Part print with two shaded views. Sizes in mm from the minimum x, y, z corner. A direction names the side the tool comes from. Coordinates: 2 decimals unless noted, no trailing zeros. Loops run counter-clockwise (first coordinate to the right, second up) from the corner with the lowest first, then second, coordinate; pieces in that order, holes last. Notation, with made-up numbers: (50.25, -12.5) -> (105.25, -12.5) arc R19 cw to (105.25, 18.5) -> close; hole circle Ø9 at (26.5, -36.75). An arc over 180 degrees is marked (long way). Use one line per item in the form item = value.
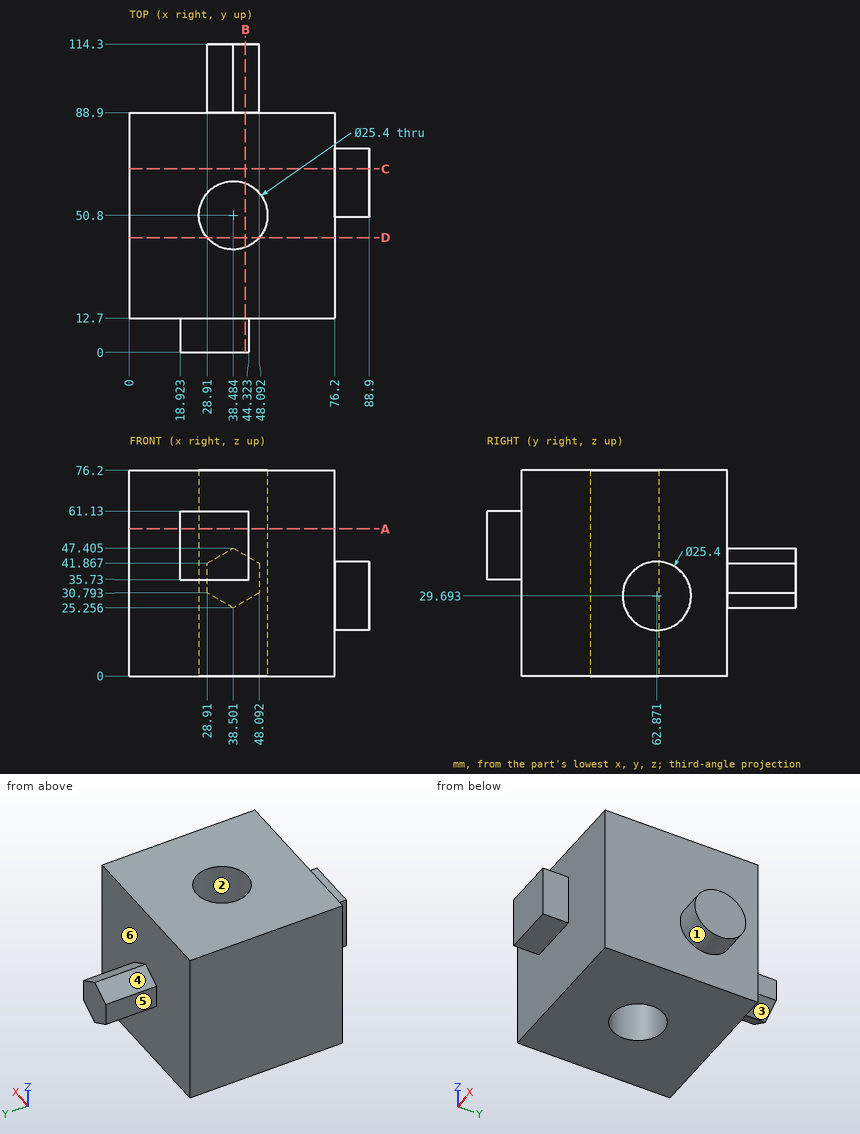
Q1. Mould opens along X. For the marked faces 1, 2 and 3 say: released by +X, released by -X, zero draft, split by the parting line, or undercut.
Result:
face_1 = zero draft
face_2 = undercut
face_3 = released by +X
Q2. Band-saw the part on B-B, the plane x = 43. Write the cut outline in (y, z).
Result:
outline = (0, 35.73) -> (12.7, 35.73) -> (12.7, 0) -> (38.93, 0) -> (38.93, 76.2) -> (12.7, 76.2) -> (12.7, 61.13) -> (0, 61.13) -> close; (62.67, 0) -> (88.9, 0) -> (88.9, 27.85) -> (114.3, 27.85) -> (114.3, 44.81) -> (88.9, 44.81) -> (88.9, 76.2) -> (62.67, 76.2) -> close
Q3. Wall check: line 1 along Y through (x, z) = (38, 42.5); line 2 along X through (y, z) = (50, 60); line 3 along X through (y, z) = (45, 72.5) (1 decimal). Give the ranges that are in metal, low to high.
Result:
line_1 = 0 to 38.11, 63.49 to 114.3
line_2 = 0 to 25.81, 51.16 to 76.2
line_3 = 0 to 27.2, 49.8 to 76.2
Q4. Which spindle directions (+Z, -Z, +X, -X, +Y, -Y) get a long thin tool onto all of the face, cutting with end or side? Do the marked faces 4, 5 and 6. Say none if no direction does.
Result:
face_4 = +Z, -X, +Y
face_5 = +Z, -Z, -X, +Y
face_6 = +Y
Q5. Band-saw the part on C-C, the plane y = 68. Write the cut outline in (x, z) (1 decimal).
Result:
outline = (0, 0) -> (76.2, 0) -> (76.2, 18.1) -> (88.9, 18.1) -> (88.9, 41.3) -> (76.2, 41.3) -> (76.2, 76.2) -> (0, 76.2) -> close
Q6. Band-saw the part on A-A, the plane z = 54.5. Write the cut outline in (x, y).
Result:
outline = (0, 12.7) -> (18.92, 12.7) -> (18.92, 0) -> (44.32, 0) -> (44.32, 12.7) -> (76.2, 12.7) -> (76.2, 88.9) -> (0, 88.9) -> close; hole circle Ø25.4 at (38.48, 50.8)
Q7. Pin check, flat tips, straight feed: pin 1 Ø5.5 at (y, z) = (103.5, 37.5) entering from +X; pin 2 Ø12 at (x, z) = (56.5, 53.5) entering from +Y; pin 3 Ø10 at (y, z) = (7, 53) entering from +X. Stop position of each tip, or through.
Result:
pin_1 = 48.09
pin_2 = 88.9
pin_3 = 44.32
Q8. Band-saw the part on D-D, the plane y = 42.5. Write the cut outline in (x, z), and give its area (3 significant figures).
Result:
outline = (0, 0) -> (28.87, 0) -> (28.87, 76.2) -> (0, 76.2) -> close; (48.1, 0) -> (76.2, 0) -> (76.2, 76.2) -> (48.1, 76.2) -> close
area = 4,340 mm2
